Design review of the part built by this model. Coordinates are the model's own, in mm. Face numbers are marked on the shaded views. A direction names the side the tool comes from. Give positions to 0.01 mm unless a question says otherwise; leave off trailing zeros. Loops run counter-clockwise (first coordinate to the right, second up) from the corner with the lowest first, then second, coordinate; pieces in that order, holes last. Notation, with made-up numbers: M 73.25,-33.75 L 130.25,-33.75 A20 ccw 130.25,-28.75 Z; hole C 35.5,57.25 d3. An arc over 180 degrees is marked long. Use CSV: the item, a comma, the result in double quotes.
from build123d import *

# Parameters (mm, degrees)
F0_W      = 25.5
F0_H      = 25.5
F0_W_2    = 20.5
F0_H_2    = 20.5
F1_DEPTH  = 35.5
F2_W      = 25.5
F2_H      = 25.5
F3_DEPTH  = 30
F4_DEPTH  = 10
F5_W      = 20.5
F5_H      = 20.5
F6_DEPTH  = 32.5
F7_W      = 20.5
F7_H      = 20.5
F8_DEPTH  = 2.5
F9_W      = 25.5
F9_H      = 25.5
F10_DEPTH = 30
F11_W     = 20.5
F11_H     = 20.5
F12_DEPTH = 32.5
F13_R     = 2.7
F14_DEPTH = 2
F15_R     = 2.7
F16_DEPTH = 2
F17_R     = 1.65
F18_DEPTH = 30
F19_R     = 2.7
F20_DEPTH = 2
F21_R     = 2.7
F22_DEPTH = 2
F23_R     = 1.65
F24_DEPTH = 30
F25_R     = 2.7
F26_DEPTH = 2
F27_R     = 1.65
F28_DEPTH = 25
F29_R     = 2.7
F30_DEPTH = 2
F31_R     = 1.65
F32_DEPTH = 25
F33_W     = 22
F33_H     = 12.5
F33_W_2   = 12.5
F33_H_2   = 22
F34_DEPTH = 2.5
F35_W     = 9.3
F35_H     = 12.5
F36_DEPTH = 2.5
F37_W     = 9.3
F37_H     = 12.5
F37_W_2   = 12.5
F37_H_2   = 12.05
F38_DEPTH = 2.5
F39_W     = 9.3
F39_H     = 12.5
F39_W_2   = 12.5
F39_H_2   = 12.05
F40_DEPTH = 2.5
F41_W     = 22
F41_H     = 12.5
F41_W_2   = 12.5
F41_H_2   = 22
F42_DEPTH = 2.5
F43_W     = 9.3
F43_H     = 12.5
F44_DEPTH = 2.5


with BuildPart() as f1:
    # F0 (on Top) → F1 (new body)
    with BuildSketch(Plane.XY):
        with Locations((0, 10.25)):
            Rectangle(F0_W, F0_H)
        with Locations((0, 10.25)):
            Rectangle(F0_W_2, F0_H_2, mode=Mode.SUBTRACT)
    extrude(amount=F1_DEPTH)

    # F2 (on face) → F3 (join)
    with BuildSketch(Plane.XZ.offset(2.5)):
        with Locations((0, 12.75)):
            Rectangle(F2_W, F2_H)
    extrude(amount=F3_DEPTH)

    # F2 (on face) → F4 (join)
    with BuildSketch(Plane.XZ.offset(2.5)):
        with Locations((0, 12.75)):
            Rectangle(F2_W, F2_H)
    extrude(amount=F4_DEPTH)

    # F5 (on face) → F6 (cut)
    with BuildSketch(Plane.XZ.offset(32.5)):
        with Locations((0, 12.75)):
            Rectangle(F5_W, F5_H)
    extrude(amount=-F6_DEPTH, mode=Mode.SUBTRACT)

    # F7 (on face) → F8 (join)
    with BuildSketch(Plane(origin=(0, 0, 0), x_dir=(1, 0, 0), z_dir=(0, 0, -1))):
        with Locations((0, -10.25)):
            Rectangle(F7_W, F7_H)
    extrude(amount=-F8_DEPTH)

    # F9 (on face) → F10 (join)
    with BuildSketch(Plane.YZ.offset(12.75)):
        with Locations((10.25, 12.75)):
            Rectangle(F9_W, F9_H)
    extrude(amount=F10_DEPTH)

    # F11 (on face) → F12 (cut)
    with BuildSketch(Plane.YZ.offset(42.75)):
        with Locations((10.25, 12.75)):
            Rectangle(F11_W, F11_H)
    extrude(amount=-F12_DEPTH, mode=Mode.SUBTRACT)

    # F13 (on face) → F14 (join)
    with BuildSketch(Plane.YZ.offset(12.75)):
        with Locations((-22.5, 12.75)):
            Circle(F13_R)
    extrude(amount=F14_DEPTH)

    # F15 (on face) → F16 (join)
    with BuildSketch(Plane(origin=(-12.75, 0, 0), x_dir=(0, -1, 0), z_dir=(-1, 0, 0))):
        with Locations((22.5, 12.75)):
            Circle(F15_R)
    extrude(amount=F16_DEPTH)

    # F17 (on face) → F18 (cut)
    with BuildSketch(Plane.YZ.offset(14.75)):
        with Locations((-22.5, 12.75)):
            Circle(F17_R)
    extrude(amount=-F18_DEPTH, mode=Mode.SUBTRACT)

    # F19 (on face) → F20 (join)
    with BuildSketch(Plane.XZ.offset(2.5)):
        with Locations((32.75, 12.75)):
            Circle(F19_R)
    extrude(amount=F20_DEPTH)

    # F21 (on face) → F22 (join)
    with BuildSketch(Plane(origin=(0, 23, 0), x_dir=(-1, 0, 0), z_dir=(0, 1, 0))):
        with Locations((-32.75, 12.75)):
            Circle(F21_R)
    extrude(amount=F22_DEPTH)

    # F23 (on face) → F24 (cut)
    with BuildSketch(Plane(origin=(0, 25, 0), x_dir=(-1, 0, 0), z_dir=(0, 1, 0))):
        with Locations((-32.75, 12.75)):
            Circle(F23_R)
    extrude(amount=-F24_DEPTH, mode=Mode.SUBTRACT)

    # F25 (on face) → F26 (join)
    with BuildSketch(Plane(origin=(-12.75, 0, 0), x_dir=(0, -1, 0), z_dir=(-1, 0, 0))):
        with Locations((-10.25, 12.75)):
            Circle(F25_R)
    extrude(amount=F26_DEPTH)

    # F27 (on face) → F28 (cut)
    with BuildSketch(Plane(origin=(-14.75, 0, 0), x_dir=(0, -1, 0), z_dir=(-1, 0, 0))):
        with Locations((-10.25, 12.75)):
            Circle(F27_R)
    extrude(amount=-F28_DEPTH, mode=Mode.SUBTRACT)

    # F29 (on face) → F30 (join)
    with BuildSketch(Plane(origin=(0, 23, 0), x_dir=(-1, 0, 0), z_dir=(0, 1, 0))):
        with Locations((0, 12.75)):
            Circle(F29_R)
    extrude(amount=F30_DEPTH)

    # F31 (on face) → F32 (cut)
    with BuildSketch(Plane(origin=(0, 25, 0), x_dir=(-1, 0, 0), z_dir=(0, 1, 0))):
        with Locations((0, 12.75)):
            Circle(F31_R)
    extrude(amount=-F32_DEPTH, mode=Mode.SUBTRACT)

    # F33 (on face) → F34 (cut)
    with BuildSketch(Plane(origin=(0, 0, 0), x_dir=(1, 0, 0), z_dir=(0, 0, -1))):
        with Locations((27.75, -10.25)):
            Rectangle(F33_W, F33_H)
        with Locations((0, -10.25)):
            Rectangle(F33_W_2, F33_H)
        with Locations((0, 17.5)):
            Rectangle(F33_W_2, F33_H_2)
    extrude(amount=-F34_DEPTH, mode=Mode.SUBTRACT)

    # F35 (on face) → F36 (cut)
    with BuildSketch(Plane.YZ.offset(12.75)):
        with Locations((-11.15, 12.75)):
            Rectangle(F35_W, F35_H)
    extrude(amount=-F36_DEPTH, mode=Mode.SUBTRACT)

    # F37 (on face) → F38 (cut)
    with BuildSketch(Plane(origin=(-12.75, 0, 0), x_dir=(0, -1, 0), z_dir=(-1, 0, 0))):
        with Locations((11.15, 12.75)):
            Rectangle(F37_W, F37_H)
        with Locations((-10.25, 25.475)):
            Rectangle(F37_W_2, F37_H_2)
    extrude(amount=-F38_DEPTH, mode=Mode.SUBTRACT)

    # F39 (on face) → F40 (cut)
    with BuildSketch(Plane(origin=(0, 23, 0), x_dir=(-1, 0, 0), z_dir=(0, 1, 0))):
        with Locations((-21.4, 12.75)):
            Rectangle(F39_W, F39_H)
        with Locations((0, 25.475)):
            Rectangle(F39_W_2, F39_H_2)
    extrude(amount=-F40_DEPTH, mode=Mode.SUBTRACT)

    # F41 (on face) → F42 (cut)
    with BuildSketch(Plane.XY.offset(25.5)):
        with Locations((27.75, 10.25)):
            Rectangle(F41_W, F41_H)
        with Locations((0, -17.5)):
            Rectangle(F41_W_2, F41_H_2)
    extrude(amount=-F42_DEPTH, mode=Mode.SUBTRACT)

    # F43 (on face) → F44 (cut)
    with BuildSketch(Plane.XZ.offset(2.5)):
        with Locations((21.4, 12.75)):
            Rectangle(F43_W, F43_H)
    extrude(amount=-F44_DEPTH, mode=Mode.SUBTRACT)


solid = f1.part
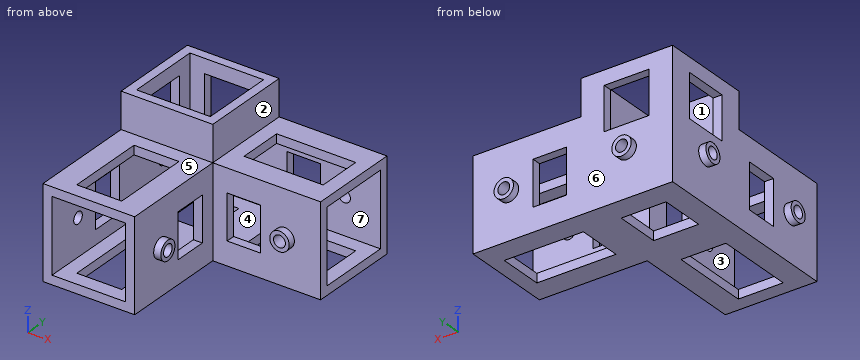
(1) Clearance check with flat-ended pins moving along their axes: P1, Ø1.5, axis at y = 13, z = 27, coming from the +X side; P2, Ø14, axis at y = 14.5, z = 26, coming from the -X side; P3, Ø13, axis at x = 34.5, y = 15.5, coming from the +Z side; P4, Ø1.6, axis at y = -22.5, z = 12, coming from the +X side. State where each tip first meets the part, or that it passes through.
A:
P1,"x = 12.75"
P2,"x = -12.75"
P3,"z = 25.5"
P4,"through"
(2) We need section D-D on y = 3. State the section outline as (x, z) points, then the cut area to 4 significant figures.
A:
outline,"M -12.75,0 L 42.75,0 L 42.75,2.5 L -10.25,2.5 L -10.25,35.5 L -12.75,35.5 Z; M 10.25,23 L 42.75,23 L 42.75,25.5 L 12.75,25.5 L 12.75,35.5 L 10.25,35.5 Z"
area,"327.5 mm²"
(3) We need section C-C on z = 21.5. State the section outline as (x, y) points, then the cut area to 3 significant figures.
A:
outline,"M -12.75,-32.5 L -10.25,-32.5 L -10.25,4 L -12.75,4 Z; M -12.75,16.5 L -10.25,16.5 L -10.25,20.5 L -6.25,20.5 L -6.25,23 L -12.75,23 Z; M 6.25,20.5 L 42.75,20.5 L 42.75,23 L 6.25,23 Z; M 10.25,-32.5 L 12.75,-32.5 L 12.75,-2.5 L 42.75,-2.5 L 42.75,0 L 10.25,0 Z"
area,"365 mm²"
(4) We need section A-A on z = 4. State the section outline as (x, y) points, then the cut area to 4 significant figures.
A:
outline,"M -12.75,-32.5 L -10.25,-32.5 L -10.25,20.5 L 42.75,20.5 L 42.75,23 L -12.75,23 Z; M 10.25,-32.5 L 12.75,-32.5 L 12.75,-2.5 L 42.75,-2.5 L 42.75,0 L 10.25,0 Z"
area,"427.5 mm²"
(5) The part is to be moulded in two halves that separate along Y. For the marked faces 4, 5, 6 and 7, say which applies: released by +Y, released by -Y, zero draft, split by the parting line, or undercut.
A:
face 4,"undercut"
face 5,"zero draft"
face 6,"released by +Y"
face 7,"undercut"
(6) We need section B-B on x = 32.75. Count the separate pieces of the cut face and the enclosed holes in it, then the cut area to 3 significant figures.
A:
separate pieces,"4"
enclosed holes,"0"
area,"159 mm²"
(7) Wall thickness on line 1 along Z through (x, y) = (0, 22); line 2 along Y through (x, z) = (-5, 25); line 3 along Y through (x, z) = (15.5, 20): over which ranges is each line inside the solid? List them lowest first. Write a range as [from, to].
A:
line 1,"[0, 11.1], [14.4, 19.45], [31.5, 35.5]"
line 2,"[-32.5, -28.5], [-6.5, 0]"
line 3,"[-2.5, 0], [20.5, 23]"
(8) Machinability: for the marked faces 1, 2 and 3, which of the approach directions +Z, -Z, +X, -X, +Y, -Y give a long, thin tool a straight path to every point of the face, cutting with its end or side? Answer none if there is none.
A:
face 1,"+Z"
face 2,"+Z, +X, +Y, -Y"
face 3,"-Y"
